Build history of the part. All positions in model axes, mm. A direction names the side the tool comes from. Coordinates: 2 decimals unless noted, no trailing zeros. Order: outer loops, then holes, each group sorted by start corner. A loop starts at its lowest first (then second) coordinate and runs counter-clockwise, first axis right, second up. Notation, with made-up numbers: (41, -6) - (90, -6) arc R10 cw to (90, 0) - close; hole circle Ø10 at (-12, 56). An arc over 180 degrees is marked (long way). One line per item, written item: value.
from build123d import *

# Parameters (mm, degrees)
BOSS_EXTRU_1_DEPTH      = 46
ENL_V_MAT_EXTRU_1_REACH = 52.942
ESQUISSE2_R             = 1.75


with BuildPart() as part:
    # Esquisse1 → Boss.-Extru.1 (new body)
    with BuildSketch(Plane(origin=(0, 0, 0), x_dir=(1, 0, 0), z_dir=(0, 1, 0))):
        Polygon((-13.6, 11.266030534), (-13.6, 0.6), (-13, 0), (13, 0), (13.6, 0.6), (13.6, 11.266030534), (16.6, 11.266030534), (16.6, -3), (-16.6, -3), (-16.6, 11.266030534), align=None)
    extrude(amount=BOSS_EXTRU_1_DEPTH)

    # Esquisse2 → Enlèv. mat.-Extru.1 (cut, up to next)
    with BuildSketch(Plane.XY.offset(3), mode=Mode.PRIVATE) as enl_v_mat_extru_1_sk1:
        with Locations((-10, 33)):
            Circle(ESQUISSE2_R)
    enl_v_mat_extru_1_tool1 = extrude(enl_v_mat_extru_1_sk1.sketch, amount=-ENL_V_MAT_EXTRU_1_REACH, mode=Mode.PRIVATE) & part.part
    # Esquisse2 → Enlèv. mat.-Extru.1 (cut, up to next)
    with BuildSketch(Plane.XY.offset(3), mode=Mode.PRIVATE) as enl_v_mat_extru_1_sk2:
        with Locations((10, 33)):
            Circle(ESQUISSE2_R)
    enl_v_mat_extru_1_tool2 = extrude(enl_v_mat_extru_1_sk2.sketch, amount=-ENL_V_MAT_EXTRU_1_REACH, mode=Mode.PRIVATE) & part.part
    # Esquisse2 → Enlèv. mat.-Extru.1 (cut, up to next)
    with BuildSketch(Plane.XY.offset(3), mode=Mode.PRIVATE) as enl_v_mat_extru_1_sk3:
        with Locations((10, 13)):
            Circle(ESQUISSE2_R)
    enl_v_mat_extru_1_tool3 = extrude(enl_v_mat_extru_1_sk3.sketch, amount=-ENL_V_MAT_EXTRU_1_REACH, mode=Mode.PRIVATE) & part.part
    # Esquisse2 → Enlèv. mat.-Extru.1 (cut, up to next)
    with BuildSketch(Plane.XY.offset(3), mode=Mode.PRIVATE) as enl_v_mat_extru_1_sk4:
        with Locations((-10, 13)):
            Circle(ESQUISSE2_R)
    enl_v_mat_extru_1_tool4 = extrude(enl_v_mat_extru_1_sk4.sketch, amount=-ENL_V_MAT_EXTRU_1_REACH, mode=Mode.PRIVATE) & part.part
    add(enl_v_mat_extru_1_tool1.solids().sort_by_distance((-10, 33, 3))[0], mode=Mode.SUBTRACT)
    add(enl_v_mat_extru_1_tool2.solids().sort_by_distance((10, 33, 3))[0], mode=Mode.SUBTRACT)
    add(enl_v_mat_extru_1_tool3.solids().sort_by_distance((10, 13, 3))[0], mode=Mode.SUBTRACT)
    add(enl_v_mat_extru_1_tool4.solids().sort_by_distance((-10, 13, 3))[0], mode=Mode.SUBTRACT)


solid = part.part
1. Band-saw the part on C-C, the plane x = 10. Give the cut face in (y, z).
Values found:
outline: (0, 0) - (11.25, 0) - (11.25, 3) - (0, 3) - close; (14.75, 0) - (31.25, 0) - (31.25, 3) - (14.75, 3) - close; (34.75, 0) - (46, 0) - (46, 3) - (34.75, 3) - close
2. Band-saw the part on D-D, the plane y = 29. Give the cut face in (x, z), and give its area (3 significant figures).
Values found:
outline: (-16.6, -11.27) - (-13.6, -11.27) - (-13.6, -0.6) - (-13, 0) - (13, 0) - (13.6, -0.6) - (13.6, -11.27) - (16.6, -11.27) - (16.6, 3) - (-16.6, 3) - close
area: 168 mm2
3. Band-saw the part on B-B, the plane z = -9.5. Give the cut face in (x, y).
Values found:
outline: (-16.6, 0) - (-13.6, 0) - (-13.6, 46) - (-16.6, 46) - close; (13.6, 0) - (16.6, 0) - (16.6, 46) - (13.6, 46) - close
4. Band-saw the part on A-A, the plane y = 13. Give the cut face in (x, z), and give its area (3 significant figures).
Values found:
outline: (-16.6, -11.27) - (-13.6, -11.27) - (-13.6, -0.6) - (-13, 0) - (-11.75, 0) - (-11.75, 3) - (-16.6, 3) - close; (-8.25, 0) - (8.25, 0) - (8.25, 3) - (-8.25, 3) - close; (11.75, 0) - (13, 0) - (13.6, -0.6) - (13.6, -11.27) - (16.6, -11.27) - (16.6, 3) - (11.75, 3) - close
area: 147 mm2
5. Flat gauge pin, fed straight in: P1, Ø5.5, axis at x = 10, y = 33, coming from the -Z side. Where does the tip first touch, or does it go through?
Values found:
P1: stops at z = 0
6. Two-plate mould, pull along Y, no slides. Class faces 1 (the face through (0, 0, 1)), 2 (the face through (13.6, 23, -6)), 3 (the face through (10.9, 34.5, 1.5)), 4 (the face through (0, 46, 1)): pulls with the +Y half, pulls with the -Y half, needs draft (parallel to the pull), parting line crosses it, or undercut.
Values found:
face 1: pulls with the -Y half
face 2: needs draft
face 3: undercut
face 4: pulls with the +Y half
7. Probe line 1 along Y through (x, z) = (10, 2.2); line 2 along X through (y, z) = (35, -7.75); line 3 along Z through (x, y) = (4, 35). List the from-to ranges inside material, lowest first.
Values found:
line 1: y = 0 to 11.25, 14.75 to 31.25, 34.75 to 46
line 2: x = -16.6 to -13.6, 13.6 to 16.6
line 3: z = 0 to 3
8. 3-axis set-ups, long thin cutter, end or side, ignore diameter. For faces 5 (the face through (0, 23, 0)), 6 (the face through (9.772, 14.735, 1.521)): which of +Z, -Z, +X, -X, +Y, -Y reach the whole face in a straight line?
Values found:
face 5: -Z, +Y, -Y
face 6: +Z, -Z
